```python
from build123d import *

# Parameters (mm, degrees)
F0_W      = 40
F0_H      = 40
F1_DEPTH  = 30
F2_T      = -2.5
F4_D      = 2.5
F5_D      = 18.5
F6_W      = 20
F6_H      = 20
F7_DEPTH  = 2.5
F9_D      = 5.5
F11_DEPTH = 0.5


with BuildPart() as f1:
    # F0 (on Top) → F1 (new body)
    with BuildSketch(Plane.XY):
        Rectangle(F0_W, F0_H)
    extrude(amount=F1_DEPTH)

    # F2
    f2_openings = [f1.faces().sort_by_distance(p)[0] for p in [
        (0, 0, 30),
    ]]
    offset(amount=F2_T, openings=f2_openings)

    # F4 (through all)
    with Locations(Plane(origin=(0, 0, 0), x_dir=(1, 0, 0), z_dir=(0, 0, -1))):
        with Locations((-11.4215728753, 11.4215728753), (11.4215728753, 11.4215728753), (-11.4215728753, -11.4215728753), (11.4215728753, -11.4215728753)):
            Hole(F4_D / 2)

    # F5 (through all)
    with Locations(Plane(origin=(0, 0, 0), x_dir=(1, 0, 0), z_dir=(0, 0, -1))):
        with Locations((0, 0)):
            Hole(F5_D / 2)

    # F6 (on face) → F7 (join)
    with BuildSketch(Plane.XZ.offset(20)):
        with Locations((-30, 10)):
            Rectangle(F6_W, F6_H)
        with Locations((30, 10)):
            Rectangle(F6_W, F6_H)
    extrude(amount=-F7_DEPTH)

    # F9 (through all)
    with Locations(Plane.XZ.offset(20)):
        with Locations((-30, 10), (30, 10)):
            Hole(F9_D / 2)

    # F10 (on face) → F11 (join)
    with BuildSketch(Plane(origin=(0, 0, 0), x_dir=(1, 0, 0), z_dir=(0, 0, -1))):
        with BuildLine():
            ThreePointArc((50, 18.75), (40.6262291254, 28.7303725924), (30.0784325835, 20))
            Line((30.0784325835, 20), (40, 20))
            Line((40, 20), (40, 17.5))
            Line((40, 17.5), (30.0784325835, 17.5))
            ThreePointArc((30.0784325835, 17.5), (40.6262291254, 8.7696274076), (50, 18.75))
        make_face()
        with BuildLine():
            Line((-40, 20), (-30.0784325835, 20))
            ThreePointArc((-30.0784325835, 20), (-50, 18.75), (-30.0784325835, 17.5))
            Line((-30.0784325835, 17.5), (-40, 17.5))
            Line((-40, 17.5), (-40, 20))
        make_face()
    extrude(amount=-F11_DEPTH)


solid = f1.part
```
Read the model definition and answer for the solid it produces. Units are mm, in the model's axes. A direction names the side the tool comes from. Give positions to 0.01 mm unless a question says otherwise; leave off trailing zeros. Write each loop counter-clockwise with the first axis right and the second up, starting at its lowest first coordinate (ties: lowest second). Pieces come first, ordered by that corner, then holes. Notation, with made-up numbers: (46.25, 44.5) - (79.25, 44.5) arc R23 cw to (79.25, 81.5) - close; hole circle Ø2 at (62.25, 7). An arc over 180 degrees is marked (long way). Write item = value, one per line. Start each with the question number.
Item 1: A tool of negligible diameter and unlimited length cuts with its end or side. For faces 5 (the flat face through (40, -19, 10)), 6 (the flat face through (-40, -19, 10)), 7 (the flat face through (-17.5, 0, 16)), 8 (the cylindrical face through (10.27, -10.94, 1.27)), 9 (the cylindrical face through (32.747, -18.732, 10.121)), from which of +Z, -Z, +X, -X, +Y, -Y can it reach the whole face along a straight path? Write none if from no direction.
Item 2: Each of these flat-tipped pins is pushed along its axis until it touches: P1, Ø9, axis at x = -30, z = 10, coming from the +Y side; P2, Ø4, axis at x = -11.42, y = 11.42, coming from the +Z side; P3, Ø1.5, axis at x = -11.42, y = -11.42, coming from the -Z side; P4, Ø10, axis at x = -0.5, y = 6, coming from the -Z side. Where does it stop, or does it pass through?
Item 3: Find section A-A (z = 23.5). Give the vertices of the cut face in (x, y), then the cut area to 3 significant figures.
Item 4: Find the intervals of material crossed by probe 1 along X at (y, z) = (-16, 2.75); probe 2 along Y at (x, z) = (37.5, 3), in increasing order. Write a range as [from, to].
Item 5: The mould has two halves that part along Y. Classify faces 1 (the flat face through (0, 17.5, 16)), 2 (the flat face through (20, 0, 15)), 3 (the flat face through (27.6, -17.5, 12.4)), 4 (the flat face through (0, -17.5, 16)): +Y half, -Y half, draft (parallel to the pull), parting line (faces both ways), or undercut.
Item 6: Find section C-C (z = 11.5). Give the vertices of the cut face in (x, y), then the cut area to 3 significant figures.
Item 7: Find section D-D (y = 7.5). Give the vertices of the cut face in (x, z).
Item 8: Find section B-B (x = 0). Give the vertices of the cut face in (y, z), then the cut area to 3 significant figures.
Response:
q1.face_5 = +Z, +X, +Y, -Y
q1.face_6 = +Z, -X, +Y, -Y
q1.face_7 = +Z
q1.face_8 = +Z, -Z
q1.face_9 = +Y, -Y
q2.P1 = -17.5
q2.P2 = 2.5
q2.P3 = through
q2.P4 = 0
q3.outline = (-20, -20) - (20, -20) - (20, 20) - (-20, 20) - close; hole (-17.5, -17.5) - (17.5, -17.5) - (17.5, 17.5) - (-17.5, 17.5) - close
q3.area = 375 mm²
q4.probe_1 = [-20, -17.5], [17.5, 20]
q4.probe_2 = [-20, -17.5]
q5.face_1 = undercut
q5.face_2 = draft
q5.face_3 = +Y half
q5.face_4 = undercut
q6.outline = (-40, -20) - (-32.3, -20) - (-32.3, -17.5) - (-40, -17.5) - close; (-27.7, -20) - (27.7, -20) - (27.7, -17.5) - (20, -17.5) - (20, 20) - (-20, 20) - (-20, -17.5) - (-27.7, -17.5) - close; (32.3, -20) - (40, -20) - (40, -17.5) - (32.3, -17.5) - close; hole (-17.5, -17.5) - (17.5, -17.5) - (17.5, 17.5) - (-17.5, 17.5) - close
q6.area = 452 mm²
q7.outline = (-20, 0) - (-5.41, 0) - (-5.41, 2.5) - (-17.5, 2.5) - (-17.5, 30) - (-20, 30) - close; (5.41, 0) - (20, 0) - (20, 30) - (17.5, 30) - (17.5, 2.5) - (5.41, 2.5) - close
q8.outline = (-20, 0) - (-9.25, 0) - (-9.25, 2.5) - (-17.5, 2.5) - (-17.5, 30) - (-20, 30) - close; (9.25, 0) - (20, 0) - (20, 30) - (17.5, 30) - (17.5, 2.5) - (9.25, 2.5) - close
q8.area = 191 mm²
